Input: part model. Units: mm. Frame: model coordinates. A direction names the side the tool comes from. Give positions to 0.01 mm unless a question says otherwise; leave off trailing zeros. Loops run counter-clockwise (first coordinate to the right, second up) from the corner with the lowest first, then second, coordinate; pieces in that order, holes last. Notation, with made-up numbers: M -30,13 L 29,13 A4 ccw 29,17 Z; hole C 47,23 d11. An arc over 180 degrees is marked long. One line per item, written item: value. Start each with the question number.
(1) Ray query, line 1 along Y through (x, z) = (-21, -1.25); line 2 along Y through (x, z) = (-24, -3.25); line 3 along Y through (x, z) = (10.5, -2.5). Return the intervals inside material, ascending. Write a range as from..to.
(2) Access query for faces 4 (the cylindrical face through (-33.21, -5.28, -6.57)), 5 (the cylindrical face through (-40.48, -117.42, -6.44)), 6 (the cylindrical face through (-33.21, -155.06, -6.13)), 7 (the flat face through (15.875, -156, -3)). Directions: +Z, -Z, +X, -X, +Y, -Y. A direction counts if a zero-diameter tool reaches every point of the face in a straight line with its end or side. Return the directions, or none.
(3) Section C-C on y = -93.5. Output: boundary loops of the cut face in (x, z) (3 decimals), plus the area to 3 significant figures.
(4) Section B-B on x = 4. Output: boundary loops of the cut face in (y, z), plus the area to 3 significant figures.
(5) Pin query (flat end, axial travel): P1, Ø6, axis at y = -136, z = -7, coming from the +X side; P2, Ø1.5, axis at x = -27, z = -1.5, coming from the +Y side; P3, Ø1.2, axis at x = 22.48, y = -153.99, coming from the +Z side; P4, Ø6, axis at y = -135, z = -3.5, coming from the -X side. Return the tip coordinate at first contact, or that it passes through.
(6) Pull-direction query (X, two-part tool) for faces 1 (the flat face through (-53.8, -72.8, -6.3)), 2 (the flat face through (-22, -156, -5.08)), 3 (the flat face through (29, -79, -12.7)); classes: released by +X, released by -X, zero draft, split by the parting line, or undercut.
(7) Section A-A on y = -33. Output: boundary loops of the cut face in (x, z) (3 decimals).
```python
from build123d import *

# Parameters (mm, degrees)
SKETCH1_W              = 12.7
SKETCH1_H              = 12.7
BOSS_EXTRUDE1_DEPTH    = 28.575
SKETCH10_W             = 12.7
SKETCH10_H             = 12.7
BOSS_EXTRUDE6_DEPTH    = 160.3375
SKETCH54_W             = 12.7
SKETCH54_H             = 12.7
BOSS_EXTRUDE10_DEPTH   = 25.4
BOSS_EXTRUDE11_DEPTH   = 12.7
F_8_32_TAPPED_HOLE11_D = 3.4544
F_8_32_TAPPED_HOLE12_D = 3.4544
SKETCH11_W             = 5.08
SKETCH11_H             = 7.9375
BOSS_EXTRUDE12_DEPTH   = 12.7
SKETCH68_W             = 6.604
SKETCH68_H             = 6.35
CUT_EXTRUDE4_DEPTH     = 1.5875
F_4_40_TAPPED_HOLE3_D  = 2.2606
SKETCH71_R             = 1.016
CUT_EXTRUDE5_DEPTH     = 1.5875
F_8_32_TAPPED_HOLE13_D = 3.4544


with BuildPart() as part:
    # Sketch1 → Boss-Extrude1 (new body)
    with BuildSketch(Plane(origin=(0, 0, 0), x_dir=(0, 0, -1), z_dir=(1, 0, 0))):
        with Locations((6.35, -6.35)):
            Rectangle(SKETCH1_W, SKETCH1_H)
    boss_extrude1 = extrude(amount=BOSS_EXTRUDE1_DEPTH)

    # Sketch10 → Boss-Extrude6 (add)
    with BuildSketch(Plane(origin=(0, 0, 0), x_dir=(1, 0, 0), z_dir=(0, 1, 0))):
        with Locations((34.925, 6.35)):
            Rectangle(SKETCH10_W, SKETCH10_H)
    boss_extrude6 = extrude(amount=-BOSS_EXTRUDE6_DEPTH)

    # Sketch54 → Boss-Extrude10 (add)
    with BuildSketch(Plane(origin=(41.275, 0, 0), x_dir=(0, 0, -1), z_dir=(1, 0, 0))):
        with Locations((6.35, -153.9875)):
            Rectangle(SKETCH54_W, SKETCH54_H)
    boss_extrude10 = extrude(amount=BOSS_EXTRUDE10_DEPTH)

    # Sketch55 → Boss-Extrude11 (add)
    with BuildSketch(Plane.XY):
        Polygon((41.275, 0), (66.675, -147.6375), (66.675, -160.3375), (28.575, -160.3375), (28.575, -12.7), (0, -12.7), (0, 0), align=None)
    boss_extrude11 = extrude(amount=-BOSS_EXTRUDE11_DEPTH)

    # Sketch56 → #8-32 Tapped Hole8 (revolve, cut)
    with BuildSketch(Plane(origin=(34.925, 0, -6.35), x_dir=(0, 0, 1), z_dir=(1, 0, 0))):
        Polygon((0, 0), (0, 11.746446461), (1.7272, 10.70864), (1.7272, 0), align=None)
    f_8_32_tapped_hole8 = revolve(axis=Axis((34.925, 6.35, -6.35), (0, -1, 0)), mode=Mode.SUBTRACT)

    # #8-32 Tapped Hole11 (through all)
    with Locations(Plane.XY):
        with Locations((41.275, -115.8875), (51.435, -134.9375)):
            f_8_32_tapped_hole11 = Hole(F_8_32_TAPPED_HOLE11_D / 2)

    # #8-32 Tapped Hole12 (through all)
    with Locations(Plane(origin=(0, 0, -12.7), x_dir=(-1, 0, 0), z_dir=(0, 0, -1))):
        with Locations((-41.275, -150.8125), (-60.325, -150.8125)):
            f_8_32_tapped_hole12 = Hole(F_8_32_TAPPED_HOLE12_D / 2)

    # Sketch11 → Boss-Extrude12 (add)
    with BuildSketch(Plane.ZY.offset(-28.575)):
        with Locations((-2.54, -156.36875)):
            Rectangle(SKETCH11_W, SKETCH11_H)
    boss_extrude12 = extrude(amount=BOSS_EXTRUDE12_DEPTH)

    # Sketch68 → Cut-Extrude4 (cut)
    with BuildSketch(Plane.XY):
        with Locations((19.177, -157.1625)):
            Rectangle(SKETCH68_W, SKETCH68_H)
    cut_extrude4 = extrude(amount=-CUT_EXTRUDE4_DEPTH, mode=Mode.SUBTRACT)

    # #4-40 Tapped Hole3 (through all)
    with Locations(Plane.XY.offset(-1.5875)):
        with Locations((18.987190852, -157.172283572)):
            f_4_40_tapped_hole3 = Hole(F_4_40_TAPPED_HOLE3_D / 2)

    # Sketch71 → Cut-Extrude5 (cut)
    with BuildSketch(Plane.XY):
        with Locations((22.479, -153.9875)):
            Circle(SKETCH71_R)
    cut_extrude5 = extrude(amount=-CUT_EXTRUDE5_DEPTH, mode=Mode.SUBTRACT)

    # Sketch76 → #8-32 Tapped Hole14 (revolve, cut)
    with BuildSketch(Plane(origin=(34.925, -160.3375, -6.35), x_dir=(0, 0, -1), z_dir=(1, 0, 0))):
        Polygon((0, 0), (0, 11.746446461), (1.7272, 10.70864), (1.7272, 0), align=None)
    f_8_32_tapped_hole14 = revolve(axis=Axis((34.925, -166.6875, -6.35), (0, 1, 0)), mode=Mode.SUBTRACT)

    # #8-32 Tapped Hole13 (through all)
    with Locations(Plane.XY):
        with Locations((51.435, -115.8875)):
            f_8_32_tapped_hole13 = Hole(F_8_32_TAPPED_HOLE13_D / 2)

    # Mirror6: Boss-Extrude1, Boss-Extrude6, Boss-Extrude10, Boss-Extrude11, #8-32 Tapped Hole8, #8-32 Tapped Hole11, #8-32 Tapped Hole12, Boss-Extrude12, Cut-Extrude4, #4-40 Tapped Hole3, Cut-Extrude5, #8-32 Tapped Hole14, #8-32 Tapped Hole13 across Right Plane
    add(boss_extrude1.mirror(Plane(origin=(0, 0, 0), x_dir=(0, 0, -1), z_dir=(1, 0, 0))))
    add(boss_extrude6.mirror(Plane(origin=(0, 0, 0), x_dir=(0, 0, -1), z_dir=(1, 0, 0))))
    add(boss_extrude10.mirror(Plane(origin=(0, 0, 0), x_dir=(0, 0, -1), z_dir=(1, 0, 0))))
    add(boss_extrude11.mirror(Plane(origin=(0, 0, 0), x_dir=(0, 0, -1), z_dir=(1, 0, 0))))
    add(f_8_32_tapped_hole8.mirror(Plane(origin=(0, 0, 0), x_dir=(0, 0, -1), z_dir=(1, 0, 0))), mode=Mode.SUBTRACT)
    add(f_8_32_tapped_hole11.mirror(Plane(origin=(0, 0, 0), x_dir=(0, 0, -1), z_dir=(1, 0, 0))), mode=Mode.SUBTRACT)
    add(f_8_32_tapped_hole12.mirror(Plane(origin=(0, 0, 0), x_dir=(0, 0, -1), z_dir=(1, 0, 0))), mode=Mode.SUBTRACT)
    add(boss_extrude12.mirror(Plane(origin=(0, 0, 0), x_dir=(0, 0, -1), z_dir=(1, 0, 0))))
    add(cut_extrude4.mirror(Plane(origin=(0, 0, 0), x_dir=(0, 0, -1), z_dir=(1, 0, 0))), mode=Mode.SUBTRACT)
    add(f_4_40_tapped_hole3.mirror(Plane(origin=(0, 0, 0), x_dir=(0, 0, -1), z_dir=(1, 0, 0))), mode=Mode.SUBTRACT)
    add(cut_extrude5.mirror(Plane(origin=(0, 0, 0), x_dir=(0, 0, -1), z_dir=(1, 0, 0))), mode=Mode.SUBTRACT)
    add(f_8_32_tapped_hole14.mirror(Plane(origin=(0, 0, 0), x_dir=(0, 0, -1), z_dir=(1, 0, 0))), mode=Mode.SUBTRACT)
    add(f_8_32_tapped_hole13.mirror(Plane(origin=(0, 0, 0), x_dir=(0, 0, -1), z_dir=(1, 0, 0))), mode=Mode.SUBTRACT)


solid = part.part
```
Output values:
1. line 1: y = -153.99..-152.4, -12.7..0
1. line 2: y = -160.34..-152.4, -12.7..0
1. line 3: y = -12.7..0
2. face 4: +Y
2. face 5: +Z, -Z
2. face 6: -Y
2. face 7: +Z, -Z, -Y
3. outline: M -57.361,-12.7 L -28.575,-12.7 L -28.575,0 L -57.361,0 Z; M 28.575,-12.7 L 57.361,-12.7 L 57.361,0 L 28.575,0 Z
3. area: 731 mm²
4. outline: M -12.7,-12.7 L 0,-12.7 L 0,0 L -12.7,0 Z
4. area: 161 mm²
5. P1: stops at x = 65.19
5. P2: stops at y = 0
5. P3: stops at z = -1.59
5. P4: stops at x = -65.02
6. face 1: released by -X
6. face 2: undercut
6. face 3: zero draft
7. outline: M -46.952,-12.7 L -28.575,-12.7 L -28.575,0 L -46.952,0 Z; M 28.575,-12.7 L 46.952,-12.7 L 46.952,0 L 28.575,0 Z
